Could you check a few things on this model? Use its own coordinates, in mm. Face numbers are marked on the shaded views. A direction names the side the tool comes from. Round coordinates to 2 decimals unless told otherwise and drop trailing zeros. Write each loop counter-clockwise with the first axis right and the second up, starting at its lowest first coordinate (ties: lowest second). Pieces come first, ordered by that corner, then holes.
```python
from build123d import *

# Parameters (mm, degrees)
PAD_DEPTH = 250


with BuildPart() as part:
    # Sketch → Pad (new body)
    with BuildSketch(Plane.YZ.offset(-125)):
        with BuildLine():
            Line((-152, -22.5), (-217, -40.001854))
            ThreePointArc((-217, 40.001854), (-242, 0), (-217, -40.001854))
            Line((-217, 40.001854), (-152, 22.5))
            Line((-152, 22.5), (-30, 22.5))
            ThreePointArc((-22.5, 30), (-26.516504, 26.516504), (-30, 22.5))
            Line((-22.5, 30), (-22.5, 152))
            Line((-22.5, 152), (-40.001854, 217))
            ThreePointArc((40.001854, 217), (0, 242), (-40.001854, 217))
            Line((40.001854, 217), (22.5, 152))
            Line((22.5, 152), (22.5, 30))
            ThreePointArc((30.00139, 22.498146), (26.517324, 26.515685), (22.5, 30))
            Line((30.00139, 22.498146), (152.00139, 22.498146))
            Line((152.00139, 22.498146), (217.00139, 40))
            ThreePointArc((217.00139, -40), (242.00139, 0), (217.00139, 40))
            Line((217.00139, -40), (152.00139, -22.498146))
            Line((152.00139, -22.498146), (30.00139, -22.498146))
            ThreePointArc((22.5, -30), (26.517324, -26.515685), (30.00139, -22.498146))
            Line((22.5, -30), (22.5, -152))
            Line((22.5, -152), (40.001854, -217))
            ThreePointArc((-40.001854, -217), (0, -242), (40.001854, -217))
            Line((-22.5, -152), (-40.001854, -217))
            Line((-22.5, -30), (-22.5, -152))
            ThreePointArc((-30, -22.5), (-26.516504, -26.516504), (-22.5, -30))
            Line((-152, -22.5), (-30, -22.5))
        make_face()
    extrude(amount=PAD_DEPTH)


solid = part.part
```
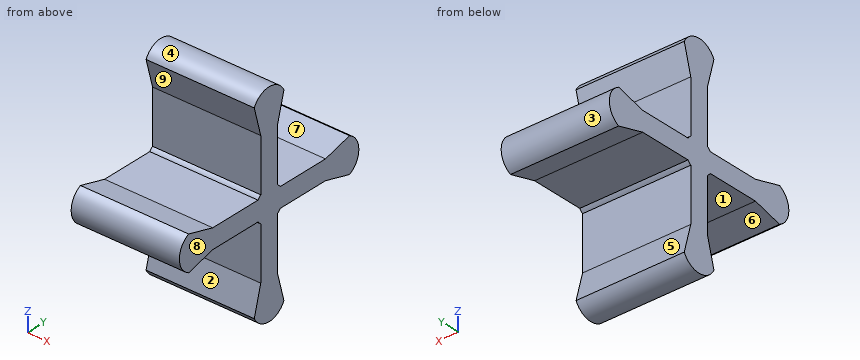
Q1. If I drill on L1, parallel to Y at x = 110, z = 40.5; L2, parallel to Z at x = -46.5, y = -2, over which ranges is the centre line in solid material (lowest first)?
Q2. On a 3-axis mill with a long thin cutter (end or side, diameter ignored), from which of +Z, -Z, +X, -X, +Y, -Y can I reach the whole of each face in a straight line? I mean the marked faces 5, 6, 7, 8 and 9. Say none if no direction works.
Q3. Imagine slicing it at A-A, the plane x = 47.5. Write out the boundary of the cut face in (y, z), then the cut area to 3 significant figures.
Q4. Imagine slicing it at C-C, the plane y = 67. Write out the boundary of the cut face in (x, z), then the cut area to 3 significant figures.
Q5. I'm going to push flat-ended pins straight in: pin 1 Ø1.5 at (x, z) = (-28, 11.5) entering from -Y; pin 2 Ø3 at (x, z) = (-97, 102) entering from -Y; pin 3 Ø1 at (x, z) = (-71, 174.5) entering from -Y. Where does each tip first touch, or does it pass through?
Q6. Imagine slicing it at B-B, the plane z = -179. Write out the boundary of the cut face in (x, y).
Q7. We'd pull the mould along Y, two halves only. Please class the marked faces 1, 2, 3 and 4: pulls with the +Y half, pulls with the -Y half, needs draft (parallel to the pull), parting line crosses it, or undercut.
Results found:
1. L1: y = -22.5 to 22.5
1. L2: z = -241.96 to 241.96
2. face 5: +X, -X, +Y
2. face 6: -Z, +X, -X
2. face 7: +Z, +X, -X
2. face 8: +Z, -Z, +X, +Y, -Y
2. face 9: +X, -X, -Y
3. outline: (-217, -40) - (-152, -22.5) - (-30, -22.5) arc R37.5 ccw to (-22.5, -30) - (-22.5, -152) - (-40, -217) arc R44.5 ccw to (40, -217) - (22.5, -152) - (22.5, -30) arc R37.5 ccw to (30, -22.5) - (152, -22.5) - (217, -40) arc R44.5 ccw to (217, 40) - (152, 22.5) - (30, 22.5) arc R37.5 ccw to (22.5, 30) - (22.5, 152) - (40, 217) arc R44.5 ccw to (-40, 217) - (-22.5, 152) - (-22.5, 30) arc R37.5 ccw to (-30, 22.5) - (-152, 22.5) - (-217, 40) arc R44.5 ccw to start
3. area: 47,400 mm2
4. outline: (-125, -22.5) - (125, -22.5) - (125, 22.5) - (-125, 22.5) - close
4. area: 11,200 mm2
5. pin 1: stops at y = -240.68
5. pin 2: stops at y = -22.5
5. pin 3: stops at y = -28.69
6. outline: (-125, -29.77) - (125, -29.77) - (125, 29.77) - (-125, 29.77) - close
7. face 1: undercut
7. face 2: pulls with the -Y half
7. face 3: pulls with the +Y half
7. face 4: parting line crosses it
